Work out the finished part from the listing and answer in its coordinate system (mm). A direction names the side the tool comes from. Round coordinates to 2 decimals unless told otherwise and drop trailing zeros. Order: outer loops, then holes, each group sorted by start corner. A loop starts at its lowest first (then second) coordinate and runs counter-clockwise, first axis right, second up. Notation, with made-up numbers: (-4.5, 76) - (32.5, 76) arc R27 cw to (32.5, 112) - close; hole circle Ø9 at (47, -21.75). An arc over 180 degrees is marked (long way). Answer in a Markdown table with one row per item.
Autodesk Inventor part; units mm, degrees
ref_plane "YZ Plane" through (0, 0, 0) normal (1, 0, 0) x (0, 1, 0)
ref_plane "XZ Plane" through (0, 0, 0) normal (0, 1, 0) x (-1, 0, 0)
ref_plane "XY Plane" through (0, 0, 0) normal (0, 0, 1) x (1, 0, 0)
sketch "Sketch1" plane through (0, 0, 0) normal (0, 1, 0) x (-1, 0, 0)
  circle A0 centre (0, 0) radius 19.1008 construction
  line L0 (0, 0) -> (113.1223, 0) construction
  circle A1 centre (113.1223, 0) radius 19.1008 construction
  line L1 (113.1223, 19.1008) -> (0, 19.1008)
  line L2 (113.1223, -19.1008) -> (0, -19.1008)
  arc A2 (113.1223, -19.1008) -> (113.1223, 19.1008) centre (113.1223, 0) ccw
  arc A3 (0, 19.1008) -> (0, -19.1008) centre (0, 0) ccw
  line L3 (0, 21.6408) -> (113.1223, 21.6408)
  arc A4 (113.1223, -21.6408) -> (113.1223, 21.6408) centre (113.1223, 0) ccw
  line L4 (113.1223, -21.6408) -> (0, -21.6408)
  arc A5 (0, 21.6408) -> (0, -21.6408) centre (0, 0) ccw
  dimension "d0" = 38.2016
  dimension "d1" = 38.2016
  dimension "d2" = 113.1223
  dimension "d3" = 2.54
extrude "Extrusion1" add sketch "Sketch1" along normal blind 9
properties part number "SHOT_1_014_Belt3" material "Rubber, Silicone"
1) The mould has two halves that part along X. Classify faces 3 (the face through (19.096, 4.437, -0.42)), 4 (the face through (-134.758, 4.437, 0.476)), 5 (the face through (-50, 9, -21)): released by +X, released by -X, zero draft, split by the parting line, or undercut.
Filled in:
| item | result |
|---|---|
| face 3 | undercut |
| face 4 | released by -X |
| face 5 | zero draft |
2) Find the intervals of material crossed by probe 1 along Z at (x, y) = (-68, 5); probe 2 along Z at (x, y) = (-127.5, 5.5); probe 3 along X at (y, z) = (1, 2), in increasing order. Write a range as from..to.
Filled in:
| item | result |
|---|---|
| probe 1 | z = -21.64..-19.1, 19.1..21.64 |
| probe 2 | z = -16.17..-12.57, 12.57..16.17 |
| probe 3 | x = -134.67..-132.12, 19..21.55 |
3) Which of the six approach directions +Z, -Z, +X, -X, +Y, -Y give full straight-line access (tool end or side, diameter ignored) to faces 1 (the face through (-57, 4, -21.641)), 2 (the face through (-57, 4, 19.101))?
Filled in:
| item | result |
|---|---|
| face 1 | -Z, +X, -X, +Y, -Y |
| face 2 | +Y, -Y |
4) This flat-tipped pin is pushed along its axis until it touches: pin 1 (1.5 mm diameter, centred on y = 1.5, z = 6, fed in from -X). Where does it stop, or does it pass through?
Filled in:
| item | result |
|---|---|
| pin 1 | stops at x = -134.12 |
5) Find section C-C, the plane z = 12. Give the vertices of the cut face in (x, y).
Filled in:
| item | result |
|---|---|
| outline | (-131.13, 0) - (-127.98, 0) - (-127.98, 9) - (-131.13, 9) - close; (14.86, 0) - (18.01, 0) - (18.01, 9) - (14.86, 9) - close |
6) Find section A-A, the plane x = -38. Give the vertices of the cut face in (y, z), then the cut area to 3 significant figures.
Filled in:
| item | result |
|---|---|
| outline | (0, -21.64) - (9, -21.64) - (9, -19.1) - (0, -19.1) - close; (0, 19.1) - (9, 19.1) - (9, 21.64) - (0, 21.64) - close |
| area | 45.7 mm^2 |
7) Find section B-B, the plane y = 3.25. Give the vertices of the cut face in (x, z), then the cut area to 3 significant figures.
Filled in:
| item | result |
|---|---|
| outline | (-113.12, -21.64) - (0, -21.64) arc R21.64 ccw to (0, 21.64) - (-113.12, 21.64) arc R21.64 ccw to start; hole (-113.12, -19.1) - (0, -19.1) arc R19.1 ccw to (0, 19.1) - (-113.12, 19.1) arc R19.1 ccw to start |
| area | 900 mm^2 |
